Input: part model. Units: mm. Frame: model coordinates. Face numbers are marked on the shaded views. A direction names the side the tool comes from. Give positions to 0.01 mm unless a question says otherwise; leave off trailing zeros. Loops run counter-clockwise (first coordinate to the right, second up) from the corner with the lowest first, then second, coordinate; pieces in that order, holes last. Notation, with made-up numbers: (-31, 73) - (-22, 73) arc R12 ccw to (-22, 89) - close; hole circle Ø9 at (6.25, -9.5). An arc over 180 degrees is marked (long way). One line per item, written item: value.
from build123d import *

# Parameters (mm, degrees)
P_IDAT_VYSUNUT_M1_DEPTH   = 15
ZAOBLIT1_R                = 7.5
SKICA6_R                  = 3.75
ODEBRAT_VYSUNUT_M4_DEPTH  = 5
SKICA7_R                  = 4.75
ODEBRAT_VYSUNUT_M5_DEPTH  = 5
P_IDAT_VYSUNUT_M2_DEPTH   = 15
SKICA10_W                 = 16.5
SKICA10_H                 = 24
ODEBRAT_VYSUNUT_M7_DEPTH  = 14
SKICA11_W                 = 2.5
SKICA11_H                 = 15
P_IDAT_VYSUNUT_M3_DEPTH   = 4
SKICA12_R                 = 0.9
ODEBRAT_VYSUNUT_M8_DEPTH  = 4
SKICA13_W                 = 4
SKICA13_H                 = 11
ODEBRAT_VYSUNUT_M9_DEPTH  = 4
SKICA15_W                 = 30.75
SKICA15_H                 = 32.5
ODEBRAT_VYSUNUT_M10_DEPTH = 30
SKICA16_R                 = 20
P_IDAT_VYSUNUT_M4_DEPTH   = 3
SKICA17_W                 = 1
SKICA17_H                 = 28
ODEBRAT_VYSUNUT_M11_DEPTH = 15
SKICA18_R                 = 6
P_IDAT_VYSUNUT_M5_DEPTH   = 0.5
SKICA19_R                 = 4.5
P_IDAT_VYSUNUT_M6_DEPTH   = 3
SKICA20_W                 = 16.5
SKICA20_H                 = 24
P_IDAT_VYSUNUT_M7_DEPTH   = 1.44
P_IDAT_VYSUNUT_M8_DEPTH   = 3
P_IDAT_START              = 1
P_IDAT_VYSUNUT_M9_DEPTH   = 1
P_IDAT_VYSUNUT_M10_DEPTH  = 3
SKICA24_R                 = 1
ODEBRAT_VYSUNUT_M12_DEPTH = 0.5
ODEBRAT_VYSUNUT_M14_DEPTH = 0.5


with BuildPart() as part:
    # Skica1 → Přidat vysunutím1 (new body)
    with BuildSketch(Plane(origin=(0, 0, 0), x_dir=(1, 0, 0), z_dir=(0, 1, 0))):
        Polygon((0, -11), (0, 11), (-3.25, 14.25), (-30.25, 14.25), (-30.25, 16.25), (-2.421572875, 16.25), (1, 12.828427125), (1, -12.828427125), (-2.421572875, -16.25), (-30.25, -16.25), (-30.25, -14.25), (-3.25, -14.25), align=None)
    extrude(amount=P_IDAT_VYSUNUT_M1_DEPTH)

    # Zaoblit1
    zaoblit1_edges = [part.edges().sort_by_distance(p)[0] for p in [
        (-30.25, 0, -15.25),
        (-30.25, 0, 15.25),
        (-30.25, 15, 15.25),
        (-30.25, 15, -15.25),
    ]]
    fillet(zaoblit1_edges, radius=ZAOBLIT1_R - 0.0001)  # a hair under: the kernel refuses the full size

    # Skica6 → Odebrat vysunutím4 (cut)
    with BuildSketch(Plane(origin=(0, 0, -16.25), x_dir=(-1, 0, 0), z_dir=(0, 0, -1))):
        with Locations((22.75, 7.5)):
            Circle(SKICA6_R)
    extrude(amount=-ODEBRAT_VYSUNUT_M4_DEPTH, mode=Mode.SUBTRACT)

    # Skica7 → Odebrat vysunutím5 (cut)
    with BuildSketch(Plane(origin=(0, 0, 14.25), x_dir=(-1, 0, 0), z_dir=(0, 0, -1))):
        with Locations((22.75, 7.5)):
            Circle(SKICA7_R)
    extrude(amount=-ODEBRAT_VYSUNUT_M5_DEPTH, mode=Mode.SUBTRACT)

    # Skica8 → Přidat vysunutím2 (add)
    with BuildSketch(Plane.XZ):
        Polygon((0.656854249, 13.171572875), (19, 13.171572875), (19, -12.828427125), (1, -12.828427125), (1, 12.828427125), align=None)
    extrude(amount=-P_IDAT_VYSUNUT_M2_DEPTH)

    # Skica10 → Odebrat vysunutím7 (cut)
    with BuildSketch(Plane(origin=(0, 15, 0), x_dir=(1, 0, 0), z_dir=(0, 1, 0))):
        with Locations((10.75, -0.171572875)):
            Rectangle(SKICA10_W, SKICA10_H)
    extrude(amount=-ODEBRAT_VYSUNUT_M7_DEPTH, mode=Mode.SUBTRACT)

    # Skica11 → Přidat vysunutím3 (add)
    with BuildSketch(Plane(origin=(19, 0, 0), x_dir=(0, 0, -1), z_dir=(1, 0, 0))):
        with Locations((-14.421572875, 7.5)):
            Rectangle(SKICA11_W, SKICA11_H)
        with Locations((14.078427125, 7.5)):
            Rectangle(SKICA11_W, SKICA11_H)
    extrude(amount=-P_IDAT_VYSUNUT_M3_DEPTH)

    # Skica12 → Odebrat vysunutím8 (cut)
    with BuildSketch(Plane(origin=(19, 0, 0), x_dir=(0, 0, -1), z_dir=(1, 0, 0))):
        with Locations((-13.671572875, 8)):
            Circle(SKICA12_R)
        with Locations((13.328427125, 8)):
            Circle(SKICA12_R)
    extrude(amount=-ODEBRAT_VYSUNUT_M8_DEPTH, mode=Mode.SUBTRACT)

    # Skica13 → Odebrat vysunutím9 (cut)
    with BuildSketch(Plane.XY.offset(13.171572875)):
        with Locations((9.156854249, 9.5)):
            Rectangle(SKICA13_W, SKICA13_H)
    extrude(amount=-ODEBRAT_VYSUNUT_M9_DEPTH, mode=Mode.SUBTRACT)

    # Skica15 → Odebrat vysunutím10 (cut)
    with BuildSketch(Plane(origin=(0, 15, 0), x_dir=(1, 0, 0), z_dir=(0, 1, 0))):
        with Locations((-14.875, 0)):
            Rectangle(SKICA15_W, SKICA15_H)
    extrude(amount=-ODEBRAT_VYSUNUT_M10_DEPTH, mode=Mode.SUBTRACT)

    # Skica16 → Přidat vysunutím4 (add)
    with BuildSketch(Plane.XZ):
        with Locations(Location((16, -5, 0), (0, 0, 92.865983983))):
            Circle(SKICA16_R)
    extrude(amount=P_IDAT_VYSUNUT_M4_DEPTH)

    # Skica17 → Odebrat vysunutím11 (cut)
    with BuildSketch(Plane(origin=(0, 15, 0), x_dir=(1, 0, 0), z_dir=(0, 1, 0))):
        with Locations((1, -0.671572875)):
            Rectangle(SKICA17_W, SKICA17_H)
    extrude(amount=-ODEBRAT_VYSUNUT_M11_DEPTH, mode=Mode.SUBTRACT)

    # Skica18 → Přidat vysunutím5 (add)
    with BuildSketch(Plane.ZY.offset(-1.5)):
        with Locations(Location((5.784090316, 7.999938585, 0), (0, 0, 180))):
            Circle(SKICA18_R)
    extrude(amount=P_IDAT_VYSUNUT_M5_DEPTH)

    # Skica19 → Přidat vysunutím6 (add)
    with BuildSketch(Plane.ZY.offset(-1)):
        with Locations((5.784090316, 7.999938585)):
            Circle(SKICA19_R)
    extrude(amount=P_IDAT_VYSUNUT_M6_DEPTH)

    # Skica20 → Přidat vysunutím7 (add)
    with BuildSketch(Plane(origin=(0, 1, 0), x_dir=(1, 0, 0), z_dir=(0, 1, 0))):
        with Locations((10.75, -0.171572875)):
            Rectangle(SKICA20_W, SKICA20_H)
    extrude(amount=P_IDAT_VYSUNUT_M7_DEPTH)

    # Skica21 → Přidat vysunutím8 (add)
    with BuildSketch(Plane(origin=(0, 0, 0), x_dir=(1, 0, 0), z_dir=(0, 1, 0))):
        with BuildLine():
            Line((29.5, 27.63922466), (31.5, 27.63922466))
            Line((31.5, 27.63922466), (31.5, 17.63922466))
            ThreePointArc((31.5, 17.63922466), (30.538588644, 18.734243344), (29.5, 19.756354563))
            Line((29.5, 19.756354563), (29.5, 27.63922466))
        make_face()
    extrude(amount=-P_IDAT_VYSUNUT_M8_DEPTH)

    # Skica22 → Přidat vysunutím9 (add)
    with BuildSketch(Plane(origin=(0, 0, 0), x_dir=(1, 0, 0), z_dir=(0, 1, 0)).offset(P_IDAT_START)):
        with BuildLine():
            Line((29.5, 27.63922466), (31.5, 27.63922466))
            Line((31.5, 27.63922466), (31.5, 17.63922466))
            ThreePointArc((31.5, 17.63922466), (33.214733837, 15.181008738), (34.542861865, 12.494149308))
            Line((34.542861865, 12.494149308), (28.646396214, 12.494149308))
            Line((28.646396214, 12.494149308), (28.646396214, 20.494149308))
            ThreePointArc((28.646396214, 20.494149308), (29.078401814, 20.131272451), (29.5, 19.756354563))
            Line((29.5, 19.756354563), (29.5, 27.63922466))
        make_face()
    extrude(amount=-P_IDAT_VYSUNUT_M9_DEPTH)

    # Skica23 → Přidat vysunutím10 (add)
    with BuildSketch(Plane.XZ):
        with BuildLine():
            Line((1.5, 8.774977314), (1.5, 13.171572875))
            Line((1.5, 13.171572875), (7.645723296, 13.171572875))
            ThreePointArc((7.645723296, 13.171572875), (4.363333637, 11.26616107), (1.5, 8.774977314))
        make_face()
    extrude(amount=P_IDAT_VYSUNUT_M10_DEPTH)

    # Skica24 → Odebrat vysunutím12 (cut)
    with BuildSketch(Plane.XZ.offset(3)):
        with Locations(Location((16, -5, 0), (0, 0, 270))):
            Circle(SKICA24_R)
    extrude(amount=-ODEBRAT_VYSUNUT_M12_DEPTH, mode=Mode.SUBTRACT)

    # Skica25 → Odebrat vysunutím14 (cut)
    with BuildSketch(Plane.XZ.offset(3)):
        Polygon((15, 7.5), (15, -4), (16, -4), (17, -4), (17, 7.5), align=None)
        Polygon((3.5, -6), (15, -6), (15, -5.000000001), (15, -4), (3.5, -4), align=None)
        Polygon((17, -5), (17, -6), (28.5, -6), (28.5, -4), (17, -4), align=None)
        Polygon((15, -6), (15, -17.5), (17, -17.5), (17, -6), (16, -6), align=None)
        with BuildLine():
            Line((15, -4), (15, -5.000000001))
            ThreePointArc((15, -5.000000001), (15.292893218, -4.292893219), (16, -4))
            Line((16, -4), (15, -4))
        make_face()
        with BuildLine():
            ThreePointArc((16, -4), (16.707106781, -4.292893219), (17, -5))
            Line((17, -5), (17, -4))
            Line((17, -4), (16, -4))
        make_face()
        with BuildLine():
            Line((16, -6), (17, -6))
            Line((17, -6), (17, -5))
            ThreePointArc((17, -5), (16.707106781, -5.707106781), (16, -6))
        make_face()
        with BuildLine():
            Line((15, -5.000000001), (15, -6))
            Line((15, -6), (16, -6))
            ThreePointArc((16, -6), (15.292893219, -5.707106782), (15, -5.000000001))
        make_face()
    extrude(amount=-ODEBRAT_VYSUNUT_M14_DEPTH, mode=Mode.SUBTRACT)


solid = part.part
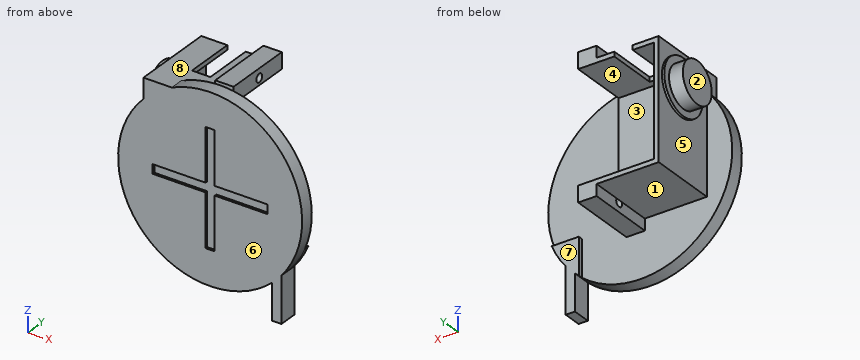
Item 1: Section A-A, the plane y = 6. Output: boundary loops of the cut face in (x, z).
Verdict:
outline: (-2, 1.75) - (1, 1.75) - (1, 0.13) - (1.5, 0.13) - (1.5, -12.83) - (15, -12.83) - (15, -15.33) - (19, -15.33) - (19, -11.83) - (2.5, -11.83) - (2.5, 12.17) - (7.16, 12.17) - (7.16, 13.17) - (1.5, 13.17) - (1.5, 11.44) - (1, 11.44) - (1, 9.82) - (-2, 9.82) - close; (11.16, 12.17) - (19, 12.17) - (19, 15.67) - (15, 15.67) - (15, 13.17) - (11.16, 13.17) - close
Item 2: Draft query along Z for the marked faces 1, 2, 3 and 4. Return one class per face: pulls with the +Z half, pulls with the -Z half, needs draft (parallel to the pull), parting line crosses it, or undercut.
Verdict:
face 1: pulls with the -Z half
face 2: needs draft
face 3: undercut
face 4: undercut
Item 3: Section B-B, the plane x = 16. Output: boundary loops of the cut face in (y, z).
Verdict:
outline: (-3, -25) - (0, -25) - (0, -15.33) - (15, -15.33) - (15, -11.83) - (2.44, -11.83) - (2.44, 12.17) - (15, 12.17) - (15, 15.67) - (0, 15.67) - (0, 15) - (-3, 15) - (-3, 7.5) - (-2.5, 7.5) - (-2.5, -17.5) - (-3, -17.5) - close; hole circle Ø1.8 at (8, -13.33); hole circle Ø1.8 at (8, 13.67)
Item 4: Pin query (flat end, axial travel): P1, Ø2, axis at x = 2, z = -19, coming from the +Y side; P2, Ø3, axis at y = 2, z = -21, coming from the +X side; P3, Ø10, axis at y = 12, z = 8, coming from the +X side. Return the tip coordinate at first contact, or that it passes through.
Verdict:
P1: stops at y = 0
P2: stops at x = 31.5
P3: stops at x = 19
Item 5: Material intervals for L1, parallel to Z at x = 6, y = 3.25; L2, parallel to Y at x = 27.5, z = 9.5; L3, parallel to X at y = 12.75, z = 13, sorted ascending.
Verdict:
L1: z = -12.83 to -11.83, 12.17 to 13.17
L2: y = -3 to 0
L3: x = 1.5 to 7.16, 11.16 to 19
Item 6: Section C-C, the plane z = -5. Output: boundary loops of the cut face in (x, y).
Verdict:
outline: (-4, -3) - (3.5, -3) - (3.5, -2.5) - (28.5, -2.5) - (28.5, -3) - (36, -3) - (36, 0) - (19, 0) - (19, 2.44) - (2.5, 2.44) - (2.5, 15) - (1.5, 15) - (1.5, 0) - (-4, 0) - close
Item 7: Section D-D, the plane x = 4. Output: boundary loops of the cut face in (y, z).
Verdict:
outline: (-3, -21) - (0, -21) - (0, -12.83) - (15, -12.83) - (15, -11.83) - (2.44, -11.83) - (2.44, 12.17) - (15, 12.17) - (15, 13.17) - (-3, 13.17) - (-3, -4) - (-2.5, -4) - (-2.5, -6) - (-3, -6) - close
Item 8: Access query for the marked faces 5, 6, 7 and 8. Directions: +Z, -Z, +X, -X, +Y, -Y. A direction counts if a zero-diameter tool reaches every point of the face in a straight line with its end or side. Return the directions, or none.
Verdict:
face 5: -X
face 6: +Z, -Z, +X, -X, -Y
face 7: +Z, -Z, +X, +Y
face 8: +Z, -X, +Y
